For this review, take the finished solid that the model builds, in its own axes (mm). A direction names the side the tool comes from. Round coordinates to 2 decimals unless told otherwise and drop trailing zeros. Order: outer loops, then holes, each group sorted by start corner. A loop starts at its lowest first (then second) coordinate and runs counter-clockwise, first axis right, second up. Notation, with made-up numbers: M -1.5,-7 L 57.5,-7 A26 cw 57.5,17 Z; hole C 74.5,28.5 d3. An arc over 180 degrees is marked long. Answer as a JSON object with one key per item and string values.
from build123d import *

# Parameters (mm, degrees)
SKETCH1_W           = 120
SKETCH1_H           = 90
SKETCH1_R           = 5
BOSS_EXTRUDE1_DEPTH = 5
SKETCH3_W           = 120
SKETCH3_H           = 90
BOSS_EXTRUDE6_DEPTH = 10
SKETCH2_R           = 12.75
CUT_EXTRUDE1_DEPTH  = 7.4
SKETCH2_8_R         = 12.75
CUT_EXTRUDE2_DEPTH  = 7.2
SKETCH2_9_R         = 12.75
CUT_EXTRUDE3_DEPTH  = 7
SKETCH2_10_R        = 12.75
CUT_EXTRUDE4_DEPTH  = 6.8
SKETCH2_11_R        = 12.75
CUT_EXTRUDE5_DEPTH  = 6.6
SKETCH2_12_R        = 12.75
CUT_EXTRUDE6_DEPTH  = 6.4
SKETCH2_13_R        = 12.75
CUT_EXTRUDE7_DEPTH  = 6.2
SKETCH2_14_R        = 12.75
CUT_EXTRUDE8_DEPTH  = 6
SKETCH2_15_R        = 12.75
CUT_EXTRUDE9_DEPTH  = 5.8
SKETCH2_16_R        = 12.75
CUT_EXTRUDE10_DEPTH = 5.6
SKETCH2_17_R        = 12.75
CUT_EXTRUDE11_DEPTH = 5.4
SKETCH2_18_R        = 12.75
CUT_EXTRUDE12_DEPTH = 5.2
SKETCH4_R           = 1.5
CUT_EXTRUDE13_DEPTH = 2


with BuildPart() as part:
    # Sketch1 → Boss-Extrude1 (new body)
    with BuildSketch(Plane(origin=(0, 0, 0), x_dir=(1, 0, 0), z_dir=(0, 1, 0))):
        Rectangle(SKETCH1_W, SKETCH1_H)
        with Locations(Location((-45, 30, 0), (0, 0, 270))):
            Circle(SKETCH1_R, mode=Mode.SUBTRACT)
        with Locations(Location((-15, 30, 0), (0, 0, 270))):
            Circle(SKETCH1_R, mode=Mode.SUBTRACT)
        with Locations(Location((15, 30, 0), (0, 0, 270))):
            Circle(SKETCH1_R, mode=Mode.SUBTRACT)
        with Locations(Location((45, 30, 0), (0, 0, 270))):
            Circle(SKETCH1_R, mode=Mode.SUBTRACT)
        with Locations(Location((-45, 0, 0), (0, 0, 270))):
            Circle(SKETCH1_R, mode=Mode.SUBTRACT)
        with Locations(Location((-15, 0, 0), (0, 0, 270))):
            Circle(SKETCH1_R, mode=Mode.SUBTRACT)
        with Locations(Location((15, 0, 0), (0, 0, 270))):
            Circle(SKETCH1_R, mode=Mode.SUBTRACT)
        with Locations(Location((45, 0, 0), (0, 0, 270))):
            Circle(SKETCH1_R, mode=Mode.SUBTRACT)
        with Locations(Location((-45, -30, 0), (0, 0, 270))):
            Circle(SKETCH1_R, mode=Mode.SUBTRACT)
        with Locations(Location((-15, -30, 0), (0, 0, 270))):
            Circle(SKETCH1_R, mode=Mode.SUBTRACT)
        with Locations(Location((15, -30, 0), (0, 0, 270))):
            Circle(SKETCH1_R, mode=Mode.SUBTRACT)
        with Locations(Location((45, -30, 0), (0, 0, 270))):
            Circle(SKETCH1_R, mode=Mode.SUBTRACT)
    extrude(amount=BOSS_EXTRUDE1_DEPTH)

    # Sketch3 → Boss-Extrude6 (add)
    with BuildSketch(Plane(origin=(0, 5, 0), x_dir=(1, 0, 0), z_dir=(0, 1, 0))):
        Rectangle(SKETCH3_W, SKETCH3_H)
    extrude(amount=BOSS_EXTRUDE6_DEPTH)

    # Sketch2 → Cut-Extrude1 (cut)
    with BuildSketch(Plane(origin=(0, 15, 0), x_dir=(1, 0, 0), z_dir=(0, 1, 0))):
        with Locations(Location((-45, 30, 0), (0, 0, 270))):
            Circle(SKETCH2_R)
    extrude(amount=-CUT_EXTRUDE1_DEPTH, mode=Mode.SUBTRACT)

    # Sketch2<8> → Cut-Extrude2 (cut)
    with BuildSketch(Plane(origin=(0, 15, 0), x_dir=(1, 0, 0), z_dir=(0, 1, 0))):
        with Locations(Location((-45, 0, 0), (0, 0, 270))):
            Circle(SKETCH2_8_R)
    extrude(amount=-CUT_EXTRUDE2_DEPTH, mode=Mode.SUBTRACT)

    # Sketch2<9> → Cut-Extrude3 (cut)
    with BuildSketch(Plane(origin=(0, 15, 0), x_dir=(1, 0, 0), z_dir=(0, 1, 0))):
        with Locations(Location((-45, -30, 0), (0, 0, 270))):
            Circle(SKETCH2_9_R)
    extrude(amount=-CUT_EXTRUDE3_DEPTH, mode=Mode.SUBTRACT)

    # Sketch2<10> → Cut-Extrude4 (cut)
    with BuildSketch(Plane(origin=(0, 15, 0), x_dir=(1, 0, 0), z_dir=(0, 1, 0))):
        with Locations(Location((-15, 30, 0), (0, 0, 270))):
            Circle(SKETCH2_10_R)
    extrude(amount=-CUT_EXTRUDE4_DEPTH, mode=Mode.SUBTRACT)

    # Sketch2<11> → Cut-Extrude5 (cut)
    with BuildSketch(Plane(origin=(0, 15, 0), x_dir=(1, 0, 0), z_dir=(0, 1, 0))):
        with Locations(Location((-15, 0, 0), (0, 0, 270))):
            Circle(SKETCH2_11_R)
    extrude(amount=-CUT_EXTRUDE5_DEPTH, mode=Mode.SUBTRACT)

    # Sketch2<12> → Cut-Extrude6 (cut)
    with BuildSketch(Plane(origin=(0, 15, 0), x_dir=(1, 0, 0), z_dir=(0, 1, 0))):
        with Locations(Location((-15, -30, 0), (0, 0, 270))):
            Circle(SKETCH2_12_R)
    extrude(amount=-CUT_EXTRUDE6_DEPTH, mode=Mode.SUBTRACT)

    # Sketch2<13> → Cut-Extrude7 (cut)
    with BuildSketch(Plane(origin=(0, 15, 0), x_dir=(1, 0, 0), z_dir=(0, 1, 0))):
        with Locations(Location((15, 30, 0), (0, 0, 270))):
            Circle(SKETCH2_13_R)
    extrude(amount=-CUT_EXTRUDE7_DEPTH, mode=Mode.SUBTRACT)

    # Sketch2<14> → Cut-Extrude8 (cut)
    with BuildSketch(Plane(origin=(0, 15, 0), x_dir=(1, 0, 0), z_dir=(0, 1, 0))):
        with Locations(Location((15, 0, 0), (0, 0, 270))):
            Circle(SKETCH2_14_R)
    extrude(amount=-CUT_EXTRUDE8_DEPTH, mode=Mode.SUBTRACT)

    # Sketch2<15> → Cut-Extrude9 (cut)
    with BuildSketch(Plane(origin=(0, 15, 0), x_dir=(1, 0, 0), z_dir=(0, 1, 0))):
        with Locations(Location((15, -30, 0), (0, 0, 270))):
            Circle(SKETCH2_15_R)
    extrude(amount=-CUT_EXTRUDE9_DEPTH, mode=Mode.SUBTRACT)

    # Sketch2<16> → Cut-Extrude10 (cut)
    with BuildSketch(Plane(origin=(0, 15, 0), x_dir=(1, 0, 0), z_dir=(0, 1, 0))):
        with Locations(Location((45, 30, 0), (0, 0, 270))):
            Circle(SKETCH2_16_R)
    extrude(amount=-CUT_EXTRUDE10_DEPTH, mode=Mode.SUBTRACT)

    # Sketch2<17> → Cut-Extrude11 (cut)
    with BuildSketch(Plane(origin=(0, 15, 0), x_dir=(1, 0, 0), z_dir=(0, 1, 0))):
        with Locations(Location((45, 0, 0), (0, 0, 270))):
            Circle(SKETCH2_17_R)
    extrude(amount=-CUT_EXTRUDE11_DEPTH, mode=Mode.SUBTRACT)

    # Sketch2<18> → Cut-Extrude12 (cut)
    with BuildSketch(Plane(origin=(0, 15, 0), x_dir=(1, 0, 0), z_dir=(0, 1, 0))):
        with Locations(Location((45, -30, 0), (0, 0, 270))):
            Circle(SKETCH2_18_R)
    extrude(amount=-CUT_EXTRUDE12_DEPTH, mode=Mode.SUBTRACT)

    # Sketch4 → Cut-Extrude13 (cut)
    with BuildSketch(Plane(origin=(0, 15, 0), x_dir=(1, 0, 0), z_dir=(0, 1, 0))):
        with Locations(Location((-57.00780573, 42.00780573, 0), (0, 0, 270))):
            Circle(SKETCH4_R)
    extrude(amount=-CUT_EXTRUDE13_DEPTH, mode=Mode.SUBTRACT)


solid = part.part
1) For L1, parallel to X at y = 11.25, z = -30; L2, parallel to X at y = 2.5, z = 1; L3, parallel to Z at x = -40.5, y = 4, list the stretches that pass through material, from the lowest coordinate up.
Geometry check:
{"L1": "x = -60 to -57.75, -32.25 to -27.75, -2.25 to 2.25, 27.75 to 32.25, 57.75 to 60", "L2": "x = -60 to -49.9, -40.1 to -19.9, -10.1 to 10.1, 19.9 to 40.1, 49.9 to 60", "L3": "z = -45 to -32.18, -27.82 to -2.18, 2.18 to 27.82, 32.18 to 45"}
2) Add section D-D on x = 24. State the section outline as (y, z) points.
Geometry check:
{"outline": "M 0,-45 L 15,-45 L 15,-39.03 L 8.8,-39.03 L 8.8,-20.97 L 15,-20.97 L 15,-9.03 L 9,-9.03 L 9,9.03 L 15,9.03 L 15,20.97 L 9.2,20.97 L 9.2,39.03 L 15,39.03 L 15,45 L 0,45 Z"}
3) Add section B-B on x = -45. State the section outline as (y, z) points.
Geometry check:
{"outline": "M 0,-45 L 15,-45 L 15,-42.75 L 7.6,-42.75 L 7.6,-17.25 L 15,-17.25 L 15,-12.75 L 7.8,-12.75 L 7.8,12.75 L 15,12.75 L 15,17.25 L 8,17.25 L 8,42.75 L 15,42.75 L 15,45 L 0,45 L 0,35 L 5,35 L 5,25 L 0,25 L 0,5 L 5,5 L 5,-5 L 0,-5 L 0,-25 L 5,-25 L 5,-35 L 0,-35 Z"}
4) Add section A-A on y = 11.75. State how many separate pieces and enclosed holes the cut face has, and give its area (3 significant figures).
Geometry check:
{"separate pieces": "1", "enclosed holes": "12", "area": "4,670 mm²"}
5) Insertion check: P1, Ø2, axis at x = -5, z = 35, coming from the -Y side; P2, Ø6, axis at x = 20.5, z = -35, coming from the +Y side; P3, Ø3, axis at x = 13.5, z = -1.5, coming from the -Y side; P4, Ø13, axis at x = 12, z = -4, coming from the +Y side. Each pin has a flat end and moves straight along its axis. Give the tip position at first contact, or say it passes through.
Geometry check:
{"P1": "stops at y = 0", "P2": "stops at y = 8.8", "P3": "stops at y = 5", "P4": "stops at y = 9"}
6) Machinability: for faces 4 (the cylindrical face through (-15, 2, 25)), 5 (the flat face through (15, 8.8, -30)), which of the approach directions +Z, -Z, +X, -X, +Y, -Y give a long, thin tool a straight path to every point of the face, cutting with its end or side? Answer none if there is none.
Geometry check:
{"face 4": "-Y", "face 5": "+Y"}
7) Mouldability with a two-part tool opening along Z and no side actions: class faces 1 (the flat face through (15, 5, 0)), 2 (the flat face through (-1, 0, -1)), 3 (the flat face through (-1, 7, 45)) as +Z half, -Z half, draft (parallel to the pull), parting line (faces both ways), or undercut.
Geometry check:
{"face 1": "undercut", "face 2": "draft", "face 3": "+Z half"}
8) Add section C-C on z = -23.5. State the section outline as (x, y) points, and give its area (3 significant figures).
Geometry check:
{"outline": "M -60,0 L 60,0 L 60,15 L 55.97,15 L 55.97,9.4 L 34.03,9.4 L 34.03,15 L 25.97,15 L 25.97,8.8 L 4.03,8.8 L 4.03,15 L -4.03,15 L -4.03,8.2 L -25.97,8.2 L -25.97,15 L -34.03,15 L -34.03,7.6 L -55.97,7.6 L -55.97,15 L -60,15 Z", "area": "1,230 mm²"}
